from build123d import *

# Parameters (mm, degrees)
BOSS_EXTRUDE4_DEPTH = 3


with BuildPart() as part:
    # Sketch1 → Boss-Extrude4 (new body)
    with BuildSketch(Plane.XY):
        with BuildLine():
            Line((-29.899423372, -36.934875117), (-23.187084604, -0.737928439))
            ThreePointArc((-23.187084604, -0.737928439), (-21.98135558, 1.701910522), (-19.676352188, 3.148823096))
            ThreePointArc((-19.676352188, 3.148823096), (0, 5.971139565), (19.676352188, 3.148823096))
            ThreePointArc((19.676352188, 3.148823096), (21.98135558, 1.701910522), (23.187084604, -0.737928439))
            Line((23.187084604, -0.737928439), (29.899423372, -36.934875117))
            ThreePointArc((29.899423372, -36.934875117), (28.093063969, -42.415981056), (22.5, -43.838335454))
            ThreePointArc((22.5, -43.838335454), (0, -40.980460744), (-22.5, -43.838335454))
            ThreePointArc((-22.5, -43.838335454), (-28.093063969, -42.415981056), (-29.899423372, -36.934875117))
        make_face()
        with BuildLine():
            Line((-19.999993368, -14.036878488), (20.000003419, -14.020845591))
            ThreePointArc((20.000003419, -14.020845591), (23.500003419, -17.520845591), (20.000003419, -21.020845591))
            Line((20.000003419, -21.020845591), (-19.999993368, -21.036878488))
            ThreePointArc((-19.999993368, -21.036878488), (-23.499993368, -17.536878488), (-19.999993368, -14.036878488))
        make_face(mode=Mode.SUBTRACT)
        with BuildLine():
            ThreePointArc((20.172628238, -2.238367072), (0, 0.971139565), (-20.172628238, -2.238367072))
            ThreePointArc((-20.172628238, -2.238367072), (-22.413590206, -6.651765928), (-18.000191351, -8.892727896))
            ThreePointArc((-18.000191351, -8.892727896), (0, -6.028860435), (18.000191351, -8.892727896))
            ThreePointArc((18.000191351, -8.892727896), (22.413590206, -6.651765928), (20.172628238, -2.238367072))
        make_face(mode=Mode.SUBTRACT)
        with BuildLine():
            ThreePointArc((22.263959391, -31.439935769), (0, -28.980460744), (-22.263959391, -31.439935769))
            ThreePointArc((-22.263959391, -31.439935769), (-24.915606249, -35.619501409), (-20.736040609, -38.271148267))
            ThreePointArc((-20.736040609, -38.271148267), (0, -35.980460744), (20.736040609, -38.271148267))
            ThreePointArc((20.736040609, -38.271148267), (24.915606249, -35.619501409), (22.263959391, -31.439935769))
        make_face(mode=Mode.SUBTRACT)
    extrude(amount=BOSS_EXTRUDE4_DEPTH)


solid = part.part
Work out the finished part from the listing and answer in its coordinate system (mm). A direction names the side the tool comes from. Give positions to 0.01 mm unless a question says otherwise; leave off trailing zeros. Loops run counter-clockwise (first coordinate to the right, second up) from the corner with the lowest first, then second, coordinate; pieces in that order, holes last. Notation, with made-up numbers: M 32,37.25 L 54,37.25 A24 cw 54,54.25 Z; hole C 80.25,47 d7. An arc over 180 degrees is marked long. Use CSV: the item, a comma, the result in double quotes.
1) Find section A-A on y = -8. Write down the section's boundary in (x, z).
Answer:
outline,"M -24.53,0 L -21.6,0 L -21.6,3 L -24.53,3 Z; M -14.99,0 L 14.99,0 L 14.99,3 L -14.99,3 Z; M 21.6,0 L 24.53,0 L 24.53,3 L 21.6,3 Z"
2) Given P1, Ø5, axis at x = -21, y = -4, coming from the -Z side; P2, Ø2, axis at x = -15.5, y = -15.5, coming from the +Z side (3 decimals); P3, Ø1.5, axis at x = 2, z = 1.5, coming from the +Y side; P4, Ø1.5, axis at x = -5, z = 1, coming from the -Y side, each flat-ended and moving along its own axis, determine where each tip first touches the part or whether it passes through.
Answer:
P1,"z = 0"
P2,"through"
P3,"y = 5.96"
P4,"y = -41.16"
3) Consider L1, parallel to Y at x = 17, z = 1.5; L2, parallel to Y at x = 3.5, z = 2.5; L3, parallel to X at y = -17, z = 2.3. Determine where each line is inside the solid, lowest interval first.
Answer:
L1,"-42.6 to -37.51, -30.41 to -21.02, -14.02 to -8.58, -1.29 to 3.88"
L2,"-41.05 to -36.04, -29.04 to -21.03, -14.03 to -6.13, 0.88 to 5.88"
L3,"-26.2 to -23.46, 23.46 to 26.2"
4) Which of the six approach directions +Z, -Z, +X, -X, +Y, -Y give full straight-line access (tool end or side, diameter ignored) to faces 4 (the cylindrical face through (-23.5, -17.6, 1.5)), 5 (the cylindrical face through (21.955, 1.73, 1.479))?
Answer:
face 4,"+Z, -Z"
face 5,"+Z, -Z, +X, +Y"
5) Determine the mould class of faces 1 (the flat face through (0, -24, 0)), 2 (the cylindrical face through (-22.437, -6.578, 1.479)), 3 (the cylindrical face through (-22.01, 1.67, 1.48)) for opening direction Y: released by +Y, released by -Y, zero draft, split by the parting line, or undercut.
Answer:
face 1,"zero draft"
face 2,"undercut"
face 3,"released by +Y"
6) Find section B-B on x = -21.5. Write down the section's boundary in (y, z), plus the area to 3 significant figures.
Answer:
outline,"M -43.59,0 L -38.36,0 L -38.36,3 L -43.59,3 Z; M -31.27,0 L -20.7,0 L -20.7,3 L -31.27,3 Z; M -14.37,0 L -8.1,0 L -8.1,3 L -14.37,3 Z; M -3.03,0 L 2.17,0 L 2.17,3 L -3.03,3 Z"
area,"81.8 mm^2"
7) Find section C-C on z = 1.8. Write down the section's boundary in (x, y), plus the area to 3 significant figures.
Answer:
outline,"M -29.9,-36.93 A6 ccw -22.5,-43.84 A90 cw 22.5,-43.84 A6 ccw 29.9,-36.93 L 23.19,-0.74 A5 ccw 19.68,3.15 A70 ccw -19.68,3.15 A5 ccw -23.19,-0.74 Z; hole M -22.26,-31.44 A3.5 ccw -20.74,-38.27 A95 cw 20.74,-38.27 A3.5 ccw 22.26,-31.44 A102 ccw Z; hole M -20.17,-2.24 A3.5 ccw -18,-8.89 A58 cw 18,-8.89 A3.5 ccw 20.17,-2.24 A65 ccw Z; hole M -20,-21.04 L 20,-21.02 A3.5 ccw 20,-14.02 L -20,-14.04 A3.5 ccw Z"
area,"1,510 mm^2"
8) Find section D-D on y = -15.5. Write down the section's boundary in (x, z).
Answer:
outline,"M -25.92,0 L -22.85,0 L -22.85,3 L -25.92,3 Z; M 22.86,0 L 25.92,0 L 25.92,3 L 22.86,3 Z"
